Here's the drawing with two shaded views (mm, measured from the low corner). I have some questions. A direction names the side the tool comes from. Give positions to 0.01 mm unless a question says otherwise; leave off trailing zeros. Write each loop counter-clockwise with the first axis right and the second up, starting at its lowest first coordinate (ties: lowest second). Pieces come first, ordered by that corner, then holes. Notation, with made-up numbers: (0, 21.5) - (42, 21.5) arc R27 ccw to (42, 54.5) - close; hole circle Ø11 at (52.5, 65). An arc over 180 degrees is marked (long way). Write item = value, one per line.
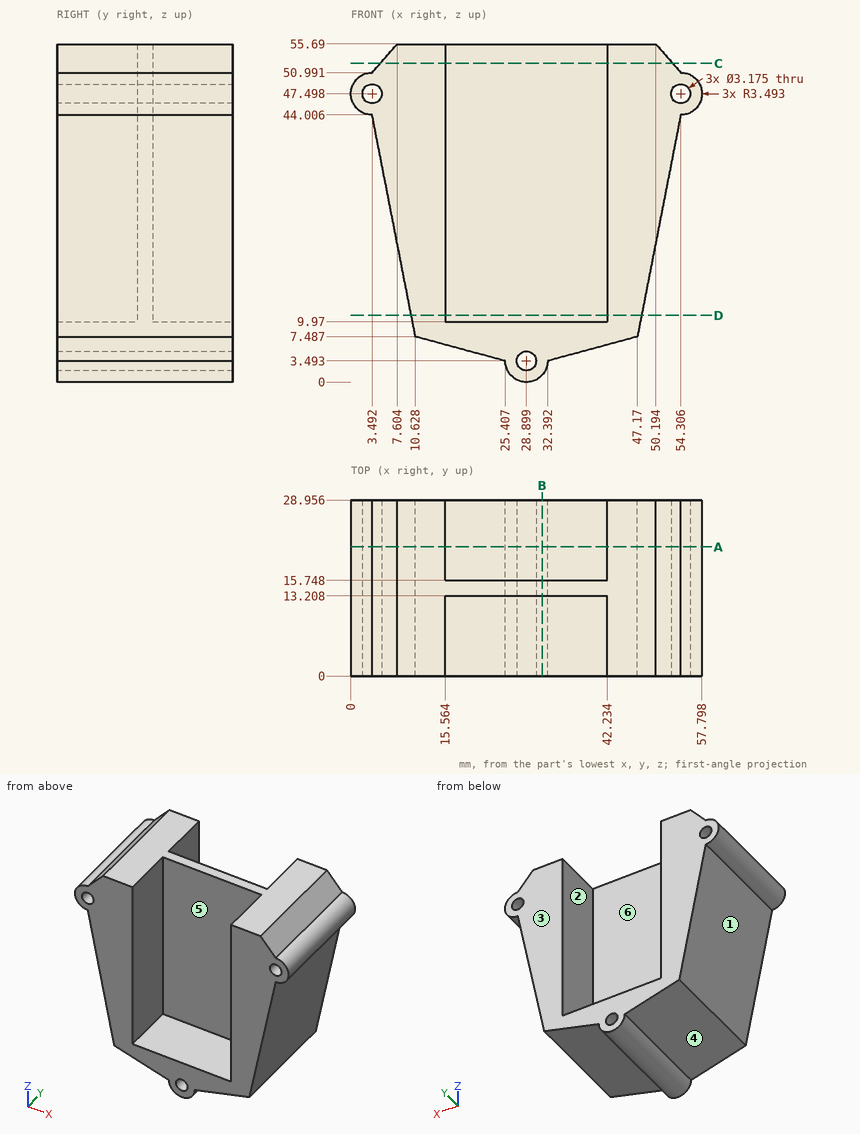
1. If we section it at B-B, the plane x = 31.5: Please give me the cut outline in (y, z) (1 decimal), and give its area (3 significant figures).
Filled sheet:
outline = (0, 1.2) - (29, 1.2) - (29, 10) - (15.7, 10) - (15.7, 55.7) - (13.2, 55.7) - (13.2, 10) - (0, 10) - close
area = 371 mm2
2. If we section it at A-A, the plane y = 21.25: Please give me the cut outline in (x, z) (1 decimal), and give its area (3 significant figures).
Filled sheet:
outline = (3.5, 44) - (10.6, 7.5) - (25.4, 3.5) arc R3.5 ccw to (32.4, 3.5) - (47.2, 7.5) - (54.3, 44) arc R3.5 ccw to (54.3, 51) - (50.2, 55.7) - (42.2, 55.7) - (42.2, 10) - (15.6, 10) - (15.6, 55.7) - (7.6, 55.7) - (3.5, 51) arc R3.5 ccw to start; hole circle Ø3.2 at (3.5, 47.5); hole circle Ø3.2 at (28.9, 3.5); hole circle Ø3.2 at (54.3, 47.5)
area = 1,070 mm2
3. Thinking about a two-plate mould opening in X: for the marked faces 1, 2 and 3, which applies, pulls with the +X half, pulls with the -X half, needs draft (parallel to the pull), parting line crosses it, or undercut?
Filled sheet:
face_1 = pulls with the -X half
face_2 = undercut
face_3 = needs draft
4. Which directions (+Z, -Z, +X, -X, +Y, -Y) give clear straight access to the entire face, cutting with the end or side of a thin tool? Please do the marked faces 4, 5 and 6.
Filled sheet:
face_4 = -Z, -X, +Y, -Y
face_5 = +Z, -Y
face_6 = +Z, +Y
5. If we section it at D-D, the plane z = 11: Please give me the cut outline in (x, y) (1 decimal).
Filled sheet:
outline = (9.9, 0) - (15.6, 0) - (15.6, 13.2) - (42.2, 13.2) - (42.2, 0) - (47.9, 0) - (47.9, 29) - (42.2, 29) - (42.2, 15.7) - (15.6, 15.7) - (15.6, 29) - (9.9, 29) - close
6. If we section it at C-C, the plane z = 52.5: Please give me the cut outline in (x, y) (1 decimal).
Filled sheet:
outline = (4.8, 0) - (15.6, 0) - (15.6, 13.2) - (42.2, 13.2) - (42.2, 0) - (53, 0) - (53, 29) - (42.2, 29) - (42.2, 15.7) - (15.6, 15.7) - (15.6, 29) - (4.8, 29) - close
7. For pin 1 (6 mm diameter, centred on y = 23, z = 30, fed in from -X); pin 2 (2 mm diameter, centred on y = 21, z = 23, fed in from +X); pin 3 (6 mm diameter, centred on x = 39, z = 23.5, fed in from -Y), each with a flat end and sliding along its axis, tell me the tip position at first contact or that it passes through.
Filled sheet:
pin_1 = 5.64
pin_2 = 50.4
pin_3 = 13.21
8. I need wall thicknesses on line 1 (X direction, y = 16, z = 48) (1 decimal); line 2 (X direction, y = 7, z = 35.5) (1 decimal); line 3 (Y direction, x = 19, z = 38). Which ranges of each line are inside material? Lowest first, please.
Filled sheet:
line_1 = 0 to 2, 5 to 15.6, 42.2 to 52.8, 55.8 to 57.8
line_2 = 5.2 to 15.6, 42.2 to 52.6
line_3 = 13.21 to 15.75
